Source: CAD feature listing. Evaluate the final solid. Frame: model axes, mm. A direction names the side the tool comes from. Give positions to 0.01 mm unless a question says otherwise; leave off trailing zeros. Loops run counter-clockwise (first coordinate to the right, second up) from the corner with the lowest first, then second, coordinate; pieces in that order, holes last. Notation, with made-up numbers: (-17, -25) -> (-3, -25) arc R14 cw to (-3, -17) -> close; hole circle Ø2 at (39, 43). An arc over 180 degrees is marked (long way). Return JSON: item names as keys, results as strings. Group by question number.
(1) Access query for faces 1 (the face through (34.63, -9.48, 1.01)), 2 (the face through (39, -6.35, 37)), 3 (the face through (-18, -9, -18)). Directions: +Z, -Z, +X, -X, +Y, -Y. A direction counts if a zero-diameter tool reaches every point of the face in a straight line with its end or side. Return the directions, or none.
(2) Cut plane C-C on z = -13. Return loops of the section in (x, y).
(3) Draft query along Y for faces 4 (the face through (-40.086, -3.131, -1.066)), 5 (the face through (-1, 0, 11)), 6 (the face through (39, -12.7, 37)), 7 (the face through (-34.72, -9.48, 1.93)). Return one class per face: released by +Y, released by -Y, zero draft, split by the parting line, or undercut.
(4) Cut plane D-D on y = -14. Return loops of the section in (x, z).
(5) Cut plane B-B on y = -8.5. Return loops of the section in (x, z), then the cut area to 3 significant figures.
(6) Pin query (flat end, axial travel): pin 1 (10 mm diameter, centred on y = -12, z = 5, fed in from -X); pin 2 (3 mm diameter, centred on y = -8.5, z = 60.5, fed in from -X); pin 3 (1 mm diameter, centred on x = -12, y = -15, fed in from +Z). Return the tip coordinate at first contact, or that it passes through.
(7) Ray query, line 1 (Y direction, x = -37.5, z = -3); line 2 (Z direction, x = 0, y = -14.75); line 3 (X direction, y = -9.5, z = 37). Return the intervals inside material, ascending. Write a range as from..to.
(8) Cut plane A-A on z = 38.1. Return loops of the section in (x, y).
```python
from build123d import *

# Parameters (mm, degrees)
SKETCH_R            = 19.84375
PAD_DEPTH           = 6.35
SKETCH001_R         = 19.84375
PAD001_DEPTH        = 6.35
LINEARPATTERN_COUNT = 2
LINEARPATTERN_PITCH = 12.7


with BuildPart() as part:
    # Sketch → Pad (new body)
    with BuildSketch(Plane.XZ):
        with BuildLine():
            ThreePointArc((44.136002, 32.82593), (0, 82.55), (-44.136002, 32.82593))
            Line((-44.136002, 32.82593), (-35.921024, -35.921024))
            Line((-35.921024, -35.921024), (0, 0))
            Line((0, 0), (35.921024, -35.921024))
            Line((35.921024, -35.921024), (44.136002, 32.82593))
        make_face()
        with Locations((0, 38.1)):
            Circle(SKETCH_R, mode=Mode.SUBTRACT)
    pad = extrude(amount=PAD_DEPTH)

    # Sketch001 (on DatumPlane) → Pad001 (join)
    with BuildSketch(Plane.XZ.offset(6.35)):
        with BuildLine():
            ThreePointArc((37.916242, 34.362546), (0, 76.2), (-37.916242, 34.362546))
            Line((-37.916242, 34.362546), (-31.430896, -31.430896))
            Line((-31.430896, -31.430896), (0, 0))
            Line((0, 0), (31.430896, -31.430896))
            Line((31.430896, -31.430896), (37.916242, 34.362546))
        make_face()
        with Locations((0, 38.1)):
            Circle(SKETCH001_R, mode=Mode.SUBTRACT)
    extrude(amount=PAD001_DEPTH)

    # LinearPattern: Pad ×2
    with Locations(*[(0, -i * LINEARPATTERN_PITCH, 0) for i in range(1, LINEARPATTERN_COUNT)]):
        add(pad)


solid = part.part
```
Answers:
{
 "1": {"face 1": "-Z, +X", "face 2": "none", "face 3": "-Z, +Y, -Y"},
 "2": {"outline": "(-38.66, -19.05) -> (-13, -19.05) -> (-13, 0) -> (-38.66, 0) -> (-38.66, -6.35) -> (-33.25, -6.35) -> (-33.25, -12.7) -> (-38.66, -12.7) -> close; (13, -19.05) -> (38.66, -19.05) -> (38.66, -12.7) -> (33.25, -12.7) -> (33.25, -6.35) -> (38.66, -6.35) -> (38.66, 0) -> (13, 0) -> close"},
 "3": {"face 4": "zero draft", "face 5": "released by +Y", "face 6": "undercut", "face 7": "undercut"},
 "4": {"outline": "(-44.14, 32.83) -> (-35.92, -35.92) -> (0, 0) -> (35.92, -35.92) -> (44.14, 32.83) arc R44.45 ccw (long way) to start; hole circle Ø39.69 at (0, 38.1)"},
 "5": {"outline": "(-37.92, 34.36) -> (-31.43, -31.43) -> (0, 0) -> (31.43, -31.43) -> (37.92, 34.36) arc R38.1 ccw (long way) to start; hole circle Ø39.69 at (0, 38.1)", "area": "4,900 mm²"},
 "6": {"pin 1": "x = -41.4", "pin 2": "x = -31.86", "pin 3": "z = 81.04"},
 "7": {"line 1": "-19.05..-12.7, -6.35..0", "line 2": "0..18.26, 57.94..82.55", "line 3": "-38.08..-19.81, 19.81..38.08"},
 "8": {"outline": "(-44.45, -19.05) -> (-19.84, -19.05) -> (-19.84, 0) -> (-44.45, 0) -> (-44.45, -6.35) -> (-38.1, -6.35) -> (-38.1, -12.7) -> (-44.45, -12.7) -> close; (19.84, -19.05) -> (44.45, -19.05) -> (44.45, -12.7) -> (38.1, -12.7) -> (38.1, -6.35) -> (44.45, -6.35) -> (44.45, 0) -> (19.84, 0) -> close"}
}
